Part model, mm, in its own coordinate system. A direction names the side the tool comes from. Give positions to 0.01 mm unless a question says otherwise; leave off trailing zeros. Order: outer loops, then holes, each group sorted by start corner. A loop starts at its lowest first (then second) coordinate and runs counter-clockwise, first axis right, second up. Notation, with made-up numbers: (81, -25) - (99, -25) arc R30 cw to (99, -2) - close; hole circle Ø2 at (55, -25). An arc over 180 degrees is marked (long way). One line per item, written item: value.
Solid Edge part; units mm, degrees
sketch "Sketch1" plane through (0, 0, 0) normal (0, -1, 0) x (1, 0, 0)
  line L0 (-130, 0) -> (-130, 15)
  line L1 (-130, 15) -> (-100, 15)
  line L2 (-100, 15) -> (-100, 25)
  line L3 (-100, 25) -> (0, 25)
  line L4 (0, 25) -> (0, 15)
  line L5 (0, 15) -> (30, 15)
  line L6 (30, 15) -> (30, 0)
  dimension "D1" = 100
revolve "RevolvedProtrusion1" add sketch "Sketch1" angle 360 about axis through (14.8745, 0, 0) along (-1, 0, 0)
properties material "Steel"
1) Slice it at D-D on x = 8.5. Write the cut outline in (y, z).
Answer:
outline: circle Ø30 at (0, 0)
2) Slice it at A-A on z = 0. Write the cut outline in (x, y).
Answer:
outline: (-130, -15) - (-100, -15) - (-100, -25) - (0, -25) - (0, -15) - (30, -15) - (30, 15) - (0, 15) - (0, 25) - (-100, 25) - (-100, 15) - (-130, 15) - close
3) Wall check: line 1 along X through (y, z) = (11, -12.5); line 2 along Y through (x, z) = (-24, 11.5); line 3 along Z through (x, y) = (-5.5, -18.5). Give the ranges that are in metal, low to high. Write a range as [from, to].
Answer:
line 1: x = [-100, 0]
line 2: y = [-22.2, 22.2]
line 3: z = [-16.82, 16.82]
4) Which spindle directions (+Z, -Z, +X, -X, +Y, -Y) get a long thin tool onto all of the face, cutting with end or side? Do faces 1 (the face through (-114.79, -0.66, -14.985)), 2 (the face through (-49.3, -7.509, 23.846)), 3 (the face through (0, -11, 11)). Say none if no direction does.
Answer:
face 1: -X
face 2: +X, -X
face 3: +X
5) Drop flat-ended pins along their axis: P1, Ø2, axis at x = -73.5, y = 13.5, coming from the +Z side; P2, Ø3, axis at y = -6.5, z = 16.5, coming from the -X side; P3, Ø1, axis at x = -8.5, z = 16, coming from the +Y side. Give the stop position or say it passes through.
Answer:
P1: stops at z = 21.65
P2: stops at x = -100
P3: stops at y = 19.62
6) Slice it at C-C on x = -43. Write the cut outline in (y, z).
Answer:
outline: circle Ø50 at (0, 0)
